from build123d import *

# Parameters (mm, degrees)
SKETCH1_R                     = 7.9375
SKETCH1_R_2                   = 3.175
BASE_FLANGE1_DEPTH            = 2.54
EDGE_FLANGE2_STRIP_W          = 11.6332
EDGE_FLANGE2_STRIP_H          = 2.54
EDGE_FLANGE2_STRIP_CUT_DEPTH  = 309.626
EDGE_FLANGE2_RELIEF_W         = 12.9032
EDGE_FLANGE2_RELIEF_H         = 1.27
EDGE_FLANGE2_RELIEF_CUT_DEPTH = 2.54
EDGE_FLANGE2_DEPTH            = 309.626


# Sheet-metal steps are written as plain solids
with BuildPart() as part:
    # Sketch1 → Base-Flange1 (new body)
    with BuildSketch(Plane(origin=(0, 0, 0), x_dir=(1, 0, 0), z_dir=(0, 1, 0))):
        with BuildLine():
            Line((109.619528436, 311.807263764), (89.361961148, 247.115522342))
            ThreePointArc((89.361961148, 247.115522342), (89.460566801, 224.034337943), (102.867006006, 205.245559798))
            ThreePointArc((102.867006006, 205.245559798), (108.478001121, 198.524407286), (110.49, 190.003314763))
            Line((110.49, 190.003314763), (110.49, 0))
            Line((110.49, 0), (-114.3, 0))
            Line((-114.3, 0), (-114.3, 336.55))
            Line((-114.3, 336.55), (-67.202083301, 336.55))
            ThreePointArc((-67.202083301, 336.55), (0, 311.15), (67.202083301, 336.55))
            Line((67.202083301, 336.55), (91.44, 336.55))
            ThreePointArc((91.44, 336.55), (106.791695758, 328.779536221), (109.619528436, 311.807263764))
        make_face()
        with Locations(Location((-86.36, 317.5, 0), (0, 0, 270))):
            Circle(SKETCH1_R, mode=Mode.SUBTRACT)
        with Locations(Location((91.44, 317.5, 0), (0, 0, 270))):
            Circle(SKETCH1_R, mode=Mode.SUBTRACT)
        with Locations(Location((91.44, 190.003314763, 0), (0, 0, 270))):
            Circle(SKETCH1_R, mode=Mode.SUBTRACT)
        with Locations(Location((-86.36, 77.503314763, 0), (0, 0, 270))):
            Circle(SKETCH1_R, mode=Mode.SUBTRACT)
        with Locations(Location((-104.900544931, 205.245559798, 0), (0, 0, 270))):
            Circle(SKETCH1_R_2, mode=Mode.SUBTRACT)
        with Locations(Location((53.876660191, 205.245559798, 0), (0, 0, 270))):
            Circle(SKETCH1_R_2, mode=Mode.SUBTRACT)
    extrude(amount=-BASE_FLANGE1_DEPTH)

    # Edge-Flange2 strip (across the edge) → Edge-Flange2 strip cut (cut)
    with BuildSketch(Plane(origin=(-114.3, -2.54, -26.924), x_dir=(1, 0, 0), z_dir=(0, 0, -1))):
        with Locations((-2.54, -1.27)):
            Rectangle(EDGE_FLANGE2_STRIP_W, EDGE_FLANGE2_STRIP_H)
    extrude(amount=EDGE_FLANGE2_STRIP_CUT_DEPTH, mode=Mode.SUBTRACT)

    # Edge-Flange2 relief (on the sheet) → Edge-Flange2 relief cut (cut)
    with BuildSketch(Plane(origin=(-111.0234, -2.54, -26.924), x_dir=(1, 0, 0), z_dir=(0, -1, 0))):
        with Locations((-5.1816, 0.635)):
            Rectangle(EDGE_FLANGE2_RELIEF_W, EDGE_FLANGE2_RELIEF_H)
    extrude(amount=-EDGE_FLANGE2_RELIEF_CUT_DEPTH, mode=Mode.SUBTRACT)

    # Edge-Flange2 section (across the edge) → Edge-Flange2 (add)
    with BuildSketch(Plane(origin=(-114.3, -2.54, -26.924), x_dir=(1, 0, 0), z_dir=(0, 0, -1))):
        with BuildLine():
            Line((0, 0.7366), (0, 25.4))
            Line((0, 25.4), (2.54, 25.4))
            Line((2.54, 25.4), (2.54, 0.7366))
            ThreePointArc((2.54, 0.7366), (2.755745145, 0.215745145), (3.2766, 0))
            Line((3.2766, 0), (3.2766, -2.54))
            ThreePointArc((3.2766, -2.54), (0.959693921, -1.580306079), (0, 0.7366))
        make_face()
    extrude(amount=EDGE_FLANGE2_DEPTH)


solid = part.part
Verification items for the finished model (mm, model axes). A direction names the side the tool comes from. Round coordinates to 2 decimals unless told otherwise and drop trailing zeros. Loops run counter-clockwise (first coordinate to the right, second up) from the corner with the lowest first, then second, coordinate; pieces in that order, holes last. Notation, with made-up numbers: (48, -10.5) - (84, -10.5) arc R18 cw to (84, -1.5) - close; hole circle Ø1 at (38, -27). An arc over 180 degrees is marked (long way). Answer in a Markdown table with one row per item. Add a question column.
Q1. Section check D-D on y = -7.5. Enter the section's corners in (x, z), plus the area to 3 significant figures.
Q2. Release check for a two-part mould opening along Z. For faces 1 (the face through (0, -2.54, -171)), 2 (the face through (91.79, -1.25, -325.43)), 3 (the face through (-98, -2, -336.55)) record: pulls with the +Z half, pulls with the -Z half, needs draft (parallel to the pull), parting line crosses it, or undercut.
Q3. Section check B-B on z = -56.5. Enter the section's corners in (x, y), plus the area to 3 significant figures.
Q4. Material ranges on line 1 (X direction, y = -9, z = -116); line 2 (Y direction, x = 22.5, z = -186.5), recorded low to high.
Q5. Tool access check on faces 4 (the face through (93.82, -1.25, -182.43)), 5 (the face through (108.422, -1.252, -198.635)), 6 (the face through (-111.76, -16, -180)). Record the directions out of +Z, -Z, +X, -X, +Y, -Y that give a thin tool (end or side, any length) a straight path to the whole face; none if there is none.
Q6. Gauge pin test, flat ends, axial feed: pin 1 (8 mm diameter, centred on x = -88.5, z = -71, fed in from -Y); pin 2 (6 mm diameter, centred on y = -17.5, z = -265, fed in from +X); pin 3 (3.5 mm diameter, centred on x = -112, y = -16, fed in from +Z). Record the tip position at first contact, or that the pin passes through.
Q7. Section check A-A on x = -86.36. Enter the section's corners in (y, z), plus the area to 3 significant figures.
Q8. Section check C-C on z = -317.5. Enter the section's corners in (x, y).
Found:
| question | item | result |
|---|---|---|
| 1 | outline | (-114.3, -336.55) - (-111.76, -336.55) - (-111.76, -26.92) - (-114.3, -26.92) - close |
| 1 | area | 786 mm² |
| 2 | face 1 | needs draft |
| 2 | face 2 | undercut |
| 2 | face 3 | pulls with the -Z half |
| 3 | outline | (-114.3, -27.94) - (-111.76, -27.94) - (-111.76, -3.28) arc R0.74 cw to (-111.02, -2.54) - (110.49, -2.54) - (110.49, 0) - (-111.02, 0) arc R3.28 ccw to (-114.3, -3.28) - close |
| 3 | area | 633 mm² |
| 4 | line 1 | x = -114.3 to -111.76 |
| 4 | line 2 | y = -2.54 to 0 |
| 5 | face 4 | +Y, -Y |
| 5 | face 5 | +X, +Y, -Y |
| 5 | face 6 | +Z, -Z, +X, -Y |
| 6 | pin 1 | stops at y = -2.54 |
| 6 | pin 2 | stops at x = -111.76 |
| 6 | pin 3 | stops at z = -26.92 |
| 7 | outline | (-2.54, -336.55) - (0, -336.55) - (0, -325.44) - (-2.54, -325.44) - close; (-2.54, -309.56) - (0, -309.56) - (0, -85.44) - (-2.54, -85.44) - close; (-2.54, -69.57) - (0, -69.57) - (0, 0) - (-2.54, 0) - close |
| 7 | area | 774 mm² |
| 8 | outline | (-114.3, -27.94) - (-111.76, -27.94) - (-111.76, -3.28) arc R0.74 cw to (-111.02, -2.54) - (-94.3, -2.54) - (-94.3, 0) - (-111.02, 0) arc R3.28 ccw to (-114.3, -3.28) - close; (-78.42, -2.54) - (-35.36, -2.54) - (-35.36, 0) - (-78.42, 0) - close; (35.36, -2.54) - (83.5, -2.54) - (83.5, 0) - (35.36, 0) - close; (99.38, -2.54) - (110.49, -2.54) - (110.49, 0) - (99.38, 0) - close |
